Build history of the part. All positions in model axes, mm. Face numbers are marked on the shaded views. A direction names the side the tool comes from. Give positions to 0.01 mm unless a question says otherwise; leave off trailing zeros. Loops run counter-clockwise (first coordinate to the right, second up) from the corner with the lowest first, then second, coordinate; pieces in that order, holes last. Notation, with made-up numbers: M -6,36 L 2,36 A16 cw 2,60 Z; hole C 5,28 d7. An arc over 180 degrees is marked long. Answer as a JSON object with one key per item and string values. Group by question number.
1. Slice it at A-A (z = -32). List the corners of the cut face in (x, y), then the cut area to 3 significant figures.
2. Drop flat-ended pins along their axis: pin 1 Ø1.5 at (x, y) = (-54, 30.5) entering from +Z; pin 2 Ø2 at (y, z) = (20.5, -30) entering from -X; pin 3 Ø8 at (x, z) = (-53, -15.5) entering from +Y. Give the stop position or say it passes through.
3. Slice it at D-D (y = 19). List the corners of the cut face in (x, z).
4. Drill centre lines: line 1 along Y through (x, z) = (-52, -19); line 2 along Y through (x, z) = (-54, -34); line 3 along Z through (x, y) = (-13, 25). Where is each one in solid material? Low to high. Write a range as [from, to].
5. Slice it at B-B (x = -12.5). List the corners of the cut face in (y, z).
6. Mould opens along Z. For the marked faces 4, 5, 6 and 7 say: released by +Z, released by -Z, zero draft, split by the parting line, or undercut.
7. Slice it at C-C (y = 32). List the corners of the cut face in (x, z).
8. 3-axis set-ups, long thin cutter, end or side, ignore diameter. For the marked faces 1, 2 and 3: which of +Z, -Z, +X, -X, +Y, -Y reach the whole face in a straight line?
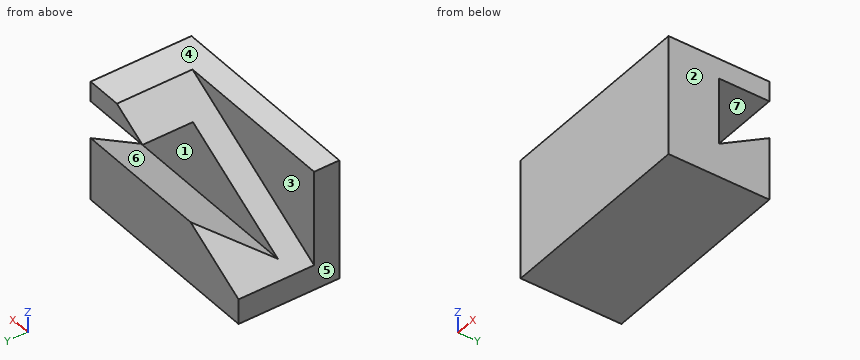
from build123d import *

# Parameters (mm, degrees)
SKIZZE1_W                       = 80
SKIZZE1_H                       = 48
AUFSATZ_LINEAR_AUSTRAGEN1_DEPTH = 40
SCHNITT_LINEAR_AUSTRAGEN1_DEPTH = 30
SCHNITT_LINEAR_AUSTRAGEN2_DEPTH = 81


with BuildPart() as part:
    # Skizze1 → Aufsatz-Linear austragen1 (new body)
    with BuildSketch(Plane(origin=(0, 0, 0), x_dir=(1, 0, 0), z_dir=(0, 1, 0))):
        with Locations((-40, 24)):
            Rectangle(SKIZZE1_W, SKIZZE1_H)
    extrude(amount=AUFSATZ_LINEAR_AUSTRAGEN1_DEPTH)

    # Skizze2 → Schnitt-Linear austragen1 (cut)
    with BuildSketch(Plane(origin=(0, 40, 0), x_dir=(1, 0, 0), z_dir=(0, 1, 0))):
        Polygon((-80, 0), (-80, 38), (-14.182069312, 0), align=None)
    extrude(amount=-SCHNITT_LINEAR_AUSTRAGEN1_DEPTH, mode=Mode.SUBTRACT)

    # Skizze4 → Schnitt-Linear austragen2 (cut, through all)
    with BuildSketch(Plane(origin=(0, 0, 0), x_dir=(0, 0, -1), z_dir=(1, 0, 0))):
        Polygon((23, 40), (34.547005384, 20), (8, 20), (8, 40), align=None)
    extrude(amount=-SCHNITT_LINEAR_AUSTRAGEN2_DEPTH, mode=Mode.SUBTRACT)


solid = part.part
Established:
{
 "1": {"outline": "M -80,0 L 0,0 L 0,20 L -69.61,20 L -69.61,10 L -80,10 Z; M -69.61,24.41 L 0,24.41 L 0,40 L -69.61,40 Z", "area": "2,580 mm^2"},
 "2": {"pin 1": "stops at z = -28.05", "pin 2": "stops at x = -67.64", "pin 3": "stops at y = 10"},
 "3": {"outline": "M -80,-48 L 0,-48 L 0,0 L -14.18,0 L -80,-38 Z"},
 "4": {"line 1": "y = [0, 10]", "line 2": "y = [0, 20], [20.95, 40]", "line 3": "z = [-48, -31.66], [-8, 0]"},
 "5": {"outline": "M 0,-48 L 40,-48 L 40,-23 L 20,-34.55 L 20,-8 L 40,-8 L 40,0 L 0,0 Z"},
 "6": {"face 4": "released by +Z", "face 5": "zero draft", "face 6": "undercut", "face 7": "undercut"},
 "7": {"outline": "M -80,-48 L 0,-48 L 0,-27.62 L -62.02,-27.62 L -80,-38 Z; M -28.04,-8 L 0,-8 L 0,0 L -14.18,0 Z"},
 "8": {"face 1": "+X, -X", "face 2": "+Z, -Z, +X, +Y, -Y", "face 3": "+Z, -X, +Y"}
}
